Geometry check sheet. Reference: the model listing, model coordinates, mm. Face numbers are marked on the shaded views. A direction names the side the tool comes from. Round coordinates to 2 decimals unless told otherwise and drop trailing zeros. Write each loop counter-clockwise with the first axis right and the second up, starting at its lowest first coordinate (ties: lowest second). Pieces come first, ordered by that corner, then holes.
Item 1: Cross-section at B-B (z = -19.2). Enter the section's corners in (x, y).
Item 2: Cross-section at C-C (z = 11.5). Enter the section's corners in (x, y), then the cut area to 3 significant figures.
Item 3: Cross-section at D-D (y = 7.5). Enter the section's corners in (x, z), then the cut area to 3 significant figures.
Item 4: Cross-section at A-A (x = 19.2). Enter the section's corners in (y, z), then the cut area to 3 significant figures.
Item 5: Scan lines: probe 1 along X at (y, z) = (2.6, -19.2); probe 2 along Y at (x, z) = (12, 21.5); probe 3 along Z at (x, y) = (20.5, 1.25). Record each from-to range of solid material in increasing order.
Item 6: Access from +Z, -Z, +X, -X, +Y, -Y to the whole of each face (thin tool, end or side, straight path). Record for the marked faces 1, 2 and 3.
Item 7: Depth check by flat-ended pin: P1, Ø1, axis at x = 17.5, y = 12, coming from the -Z side; P2, Ø1, axis at y = 10.5, z = -12, coming from the +X side; P3, Ø8, axis at x = -6, y = 10, coming from the +Z side. Enter the tip coordinate at first touch or a pass-through.
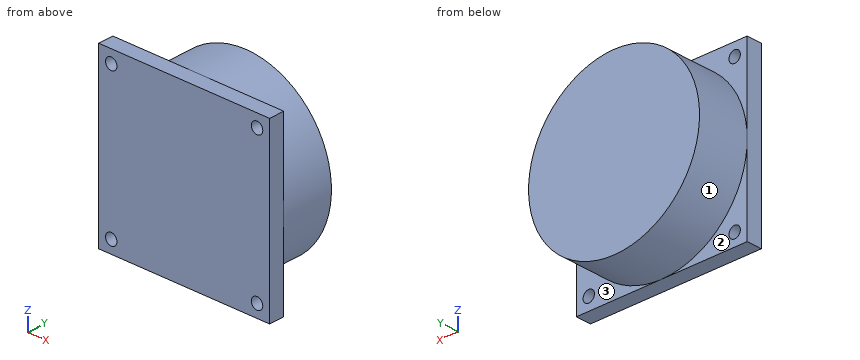
from build123d import *

# Parameters (mm, degrees)
SKETCH_1_R      = 1.5
SKETCH_1_R_2    = 22.5
EXTRUDE_1_DEPTH = 4
SKETCH_1_3_R    = 22.5
EXTRUDE_2_DEPTH = 17.5


with BuildPart() as part:
    # Sketch 1 → Extrude 1 (new body)
    # profile 1 of 5: a face of its own
    with BuildSketch(Plane(origin=(0, 0, 0), x_dir=(1, 0, 0), z_dir=(0, 1, 0))):
        with BuildLine():
            ThreePointArc((5e-08, -22.5), (-15.909902568, -15.909902586), (-22.5, 2.4e-08))
            Line((-22.5, 2.4e-08), (-22.5, -22.5))
            Line((-22.5, -22.5), (5e-08, -22.5))
        make_face()
        with Locations(Location((-19.2, -19.2, 0), (0, 0, 270))):
            Circle(SKETCH_1_R, mode=Mode.SUBTRACT)
    # profile 2 of 5: a face of its own
    with BuildSketch(Plane(origin=(0, 0, 0), x_dir=(1, 0, 0), z_dir=(0, 1, 0))):
        with BuildLine():
            Line((2.5e-08, 22.5), (-22.5, 22.5))
            Line((-22.5, 22.5), (-22.5, 2.4e-08))
            ThreePointArc((-22.5, 2.4e-08), (-15.909902559, 15.909902594), (2.5e-08, 22.5))
        make_face()
        with Locations(Location((-19.2, 19.2, 0), (0, 0, 270))):
            Circle(SKETCH_1_R, mode=Mode.SUBTRACT)
    # profile 3 of 5: a face of its own
    with BuildSketch(Plane(origin=(0, 0, 0), x_dir=(1, 0, 0), z_dir=(0, 1, 0))):
        with BuildLine():
            Line((22.5, 22.5), (2.5e-08, 22.5))
            ThreePointArc((2.5e-08, 22.5), (15.909902585, 15.909902568), (22.5, 0))
            Line((22.5, 0), (22.5, 22.5))
        make_face()
        with Locations(Location((19.2, 19.2, 0), (0, 0, 270))):
            Circle(SKETCH_1_R, mode=Mode.SUBTRACT)
    # profile 4 of 5: a face of its own
    with BuildSketch(Plane(origin=(0, 0, 0), x_dir=(1, 0, 0), z_dir=(0, 1, 0))):
        Circle(SKETCH_1_R_2)
    # profile 5 of 5: a face of its own
    with BuildSketch(Plane(origin=(0, 0, 0), x_dir=(1, 0, 0), z_dir=(0, 1, 0))):
        with BuildLine():
            Line((22.5, -22.5), (22.5, 0))
            ThreePointArc((22.5, 0), (15.909902594, -15.909902559), (5e-08, -22.5))
            Line((5e-08, -22.5), (22.5, -22.5))
        make_face()
        with Locations(Location((19.2, -19.2, 0), (0, 0, 270))):
            Circle(SKETCH_1_R, mode=Mode.SUBTRACT)
    extrude(amount=EXTRUDE_1_DEPTH)

    # Sketch 1_3 → Extrude 2 (add)
    with BuildSketch(Plane(origin=(0, 0, 0), x_dir=(1, 0, 0), z_dir=(0, 1, 0))):
        with Locations(Location((0, 0, 0), (0, 0, 270))):
            Circle(SKETCH_1_3_R)
    extrude(amount=EXTRUDE_2_DEPTH)


solid = part.part
Resolved:
1. outline: (-22.5, 0) - (-20.7, 0) - (-20.7, 4) - (-22.5, 4) - close; (-17.7, 0) - (17.7, 0) - (17.7, 4) - (11.73, 4) - (11.73, 17.5) - (-11.73, 17.5) - (-11.73, 4) - (-17.7, 4) - close; (20.7, 0) - (22.5, 0) - (22.5, 4) - (20.7, 4) - close
2. outline: (-22.5, 0) - (22.5, 0) - (22.5, 4) - (19.34, 4) - (19.34, 17.5) - (-19.34, 17.5) - (-19.34, 4) - (-22.5, 4) - close
2. area: 702 mm2
3. outline: circle Ø45 at (0, 0)
3. area: 1,590 mm2
4. outline: (0, -22.5) - (4, -22.5) - (4, -20.7) - (0, -20.7) - close; (0, -17.7) - (4, -17.7) - (4, -11.73) - (17.5, -11.73) - (17.5, 11.73) - (4, 11.73) - (4, 17.7) - (0, 17.7) - close; (0, 20.7) - (4, 20.7) - (4, 22.5) - (0, 22.5) - close
4. area: 473 mm2
5. probe 1: x = -22.5 to -20.7, -17.7 to 17.7, 20.7 to 22.5
5. probe 2: y = 0 to 4
5. probe 3: z = -22.5 to -19.95, -18.45 to 18.45, 19.95 to 22.5
6. face 1: +Y
6. face 2: -Z, -X, +Y
6. face 3: -Z, +X, +Y
7. P1: stops at z = -14.74
7. P2: stops at x = 19.34
7. P3: stops at z = 22.41
